CAD build for the part. Positions are in the model's coordinates, mm. Round coordinates to 2 decimals unless told otherwise and drop trailing zeros. Write each loop counter-clockwise with the first axis right and the second up, starting at its lowest first coordinate (ties: lowest second). Pieces come first, ordered by that corner, then holes. Notation, with made-up numbers: (10, 13) - (58, 13) arc R34 ccw to (58, 52) - close; hole circle Ø6 at (22, 29.25). An arc over 180 degrees is marked (long way). Answer in a Markdown table with one row per item.
```python
from build123d import *

# Parameters (mm, degrees)
SKETCH001_R  = 3.8
PAD001_DEPTH = 20
SKETCH_R     = 4
PAD_DEPTH    = 10


with BuildPart() as rodmount:
    # Sketch001 → Pad001 (new body)
    with BuildSketch(Plane.XZ.offset(10)):
        with Locations((0, 10)):
            Circle(SKETCH001_R)
    extrude(amount=-PAD001_DEPTH)


with BuildPart() as rodmount001:
    # Sketch → Pad (new body)
    with BuildSketch(Plane.YZ):
        with BuildLine():
            ThreePointArc((-10, 4.2e-05), (-2.1e-05, -10), (10, 0))
            Line((10, 15.000042), (10, 0))
            Line((-10, 15.000042), (10, 15.000042))
            Line((-10, 4.2e-05), (-10, 15.000042))
        make_face()
        Circle(SKETCH_R, mode=Mode.SUBTRACT)
    extrude(amount=PAD_DEPTH)

    # Cut: cut RodMount
    add(rodmount.part, mode=Mode.SUBTRACT)


solid = rodmount001.part
```
Q1. Saw through at A-A on y = 0. List the corners of the cut face in (x, z), then the cut area to 3 significant figures.
Computed:
| item | result |
|---|---|
| outline | (0, -10) - (10, -10) - (10, -4) - (0, -4) - close; (0, 4) - (10, 4) - (10, 15) - (0, 15) - (0, 13.8) arc R3.8 cw to (0, 6.2) - close |
| area | 147 mm2 |
Q2. Saw through at C-C on x = 6.25. List the corners of the cut face in (y, z), then the cut area to 3 significant figures.
Computed:
| item | result |
|---|---|
| outline | (-10, 0) arc R10 ccw to (10, 0) - (10, 15) - (-10, 15) - close; hole circle Ø8 at (0, 0) |
| area | 407 mm2 |
Q3. Saw through at D-D on x = 2. List the corners of the cut face in (y, z).
Computed:
| item | result |
|---|---|
| outline | (-10, 0) arc R10 ccw to (10, 0) - (10, 6.77) - (-10, 6.77) - close; (-10, 13.23) - (10, 13.23) - (10, 15) - (-10, 15) - close; hole circle Ø8 at (0, 0) |
Q4. Pull direction Z, two halves, no side cores. Call faces 1 (the flat face through (5, 0, 15)), 2 (the cylindrical face through (3.8, -0.1, 9.9)), 3 (the flat face through (0, 0, 14)): released by +Z, released by -Z, zero draft, split by the parting line, or undercut.
Computed:
| item | result |
|---|---|
| face 1 | released by +Z |
| face 2 | undercut |
| face 3 | zero draft |
Q5. Drill centre lines: line 1 (Z direction, x = 4, y = 0); line 2 (Z direction, x = 2.25, y = -0.25); line 3 (Z direction, x = 1, y = -0.75). Where is each one in solid material? Low to high.
Computed:
| item | result |
|---|---|
| line 1 | z = -10 to -4, 4 to 15 |
| line 2 | z = -10 to -3.99, 3.99 to 6.94, 13.06 to 15 |
| line 3 | z = -9.97 to -3.93, 3.93 to 6.33, 13.67 to 15 |
Q6. Flat gauge pins, fed straight in: pin 1 (1.5 mm diameter, centred on y = -7.5, z = 10.5, fed in from -X); pin 2 (5 mm diameter, centred on y = 0, z = 0, fed in from +X). Where does each tip first touch, or does it go through?
Computed:
| item | result |
|---|---|
| pin 1 | stops at x = 3.59 |
| pin 2 | passes through |
Q7. Saw through at B-B on z = -3. List the corners of the cut face in (x, y).
Computed:
| item | result |
|---|---|
| outline | (0, -9.54) - (10, -9.54) - (10, -2.65) - (0, -2.65) - close; (0, 2.65) - (10, 2.65) - (10, 9.54) - (0, 9.54) - close |
